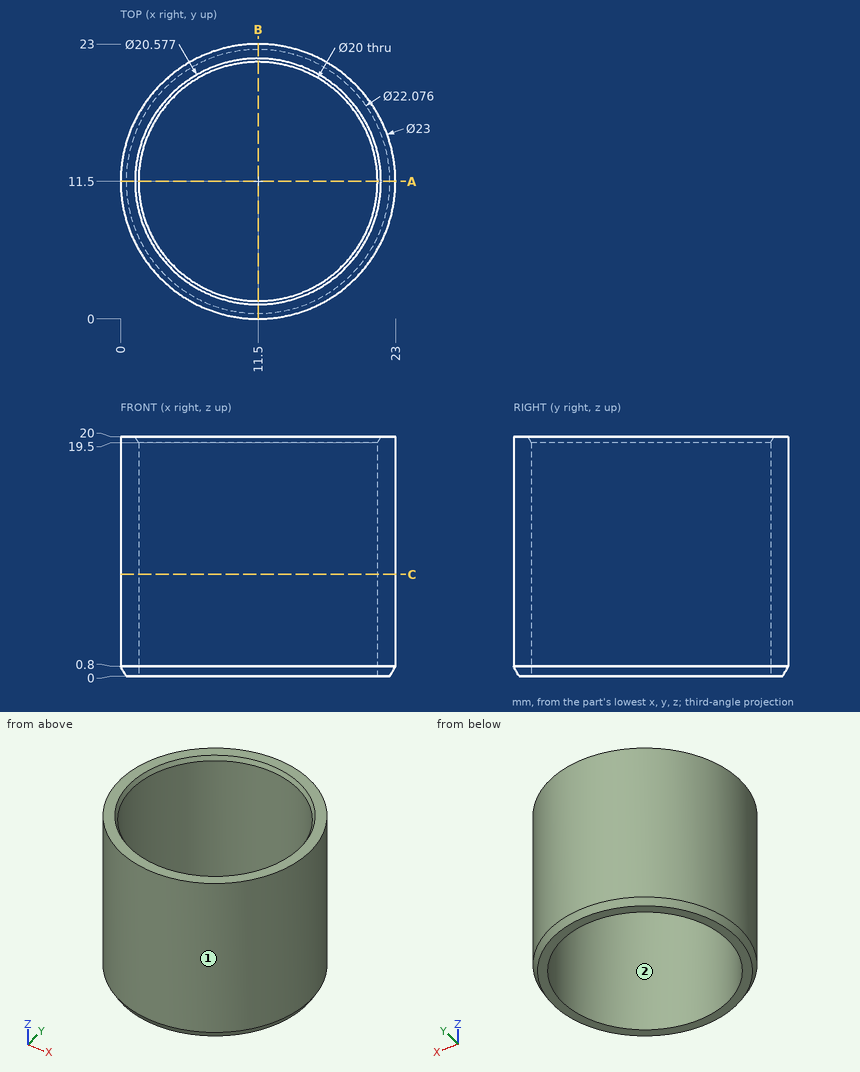
Check sheet for the drawn part. Datum: minimum x, y, z corner. Units: mm. Give positions to 0.01 mm unless a question says otherwise; leave off trailing zeros. Write each loop counter-clockwise with the first axis right and the second up, starting at its lowest first coordinate (ties: lowest second). Pieces come first, ordered by that corner, then holes.
(1) Material ranges on line 1 (Y direction, x = 11.5, z = 7.75); line 2 (X direction, y = 20.25, z = 15.25) (1 decimal); line 3 (Y direction, x = 6.5, z = 8) (1 decimal), recorded low to high.
(2) Cross-section at C-C (z = 8.5). Enter the section's corners in (x, y), plus the area to 3 significant figures.
(3) Cross-section at A-A (y = 11.5). Enter the section's corners in (x, z).
(4) Gauge pin test, flat ends, axial feed: pin 1 (2 mm diameter, centred on x = 17.5, z = 3, fed in from -Y); pin 2 (4 mm diameter, centred on y = 9, z = 11.5, fed in from +X); pin 3 (8 mm diameter, centred on y = 3.5, z = 3.5, fed in from +X); pin 4 (5 mm diameter, centred on x = 18, y = 12.5, fed in from -Z). Record the tip position at first contact, or that the pin passes through.
(5) Mould release check, pull along Y, two halves, no side actions. Record for the marked faces 1 and 2: +Y half, -Y half, draft (parallel to the pull), parting line (faces both ways), or undercut.
Worked out:
1. line 1: y = 0 to 1.5, 21.5 to 23
1. line 2: x = 4 to 6.7, 16.3 to 19
1. line 3: y = 1.1 to 2.8, 20.2 to 21.9
2. outline: circle Ø23 at (11.5, 11.5); hole circle Ø20 at (11.5, 11.5)
2. area: 101 mm2
3. outline: (0, 0.8) - (0.46, 0) - (1.5, 0) - (1.5, 19.5) - (1.21, 20) - (0, 20) - close; (21.5, 0) - (22.54, 0) - (23, 0.8) - (23, 20) - (21.79, 20) - (21.5, 19.5) - close
4. pin 1: stops at y = 1.14
4. pin 2: stops at x = 22.99
4. pin 3: stops at x = 22.28
4. pin 4: passes through
5. face 1: parting line
5. face 2: undercut
